```python
from build123d import *

# Parameters (mm, degrees)
SALIENTE_EXTRUIR1_DEPTH = 8
CORTAR_EXTRUIR1_DEPTH   = 10


with BuildPart() as part:
    # Croquis2 → Saliente-Extruir1 (new body)
    with BuildSketch(Plane.XY):
        with BuildLine():
            Line((614.835603051, 709.114300051), (830.835603051, 709.114300051))
            ThreePointArc((830.835603051, 709.114300051), (835.078243738, 710.871659363), (836.835603051, 715.114300051))
            Line((836.835603051, 715.114300051), (836.835603051, 819.114300051))
            ThreePointArc((836.835603051, 819.114300051), (835.078243738, 823.356940738), (830.835603051, 825.114300051))
            Line((830.835603051, 825.114300051), (614.835603051, 825.114300051))
            ThreePointArc((614.835603051, 825.114300051), (610.592962364, 823.356940738), (608.835603051, 819.114300051))
            Line((608.835603051, 819.114300051), (608.835603051, 715.114300051))
            ThreePointArc((608.835603051, 715.114300051), (610.592962364, 710.871659363), (614.835603051, 709.114300051))
        make_face()
    extrude(amount=SALIENTE_EXTRUIR1_DEPTH)

    # Croquis3 → Cortar-Extruir1 (cut)
    with BuildSketch(Plane(origin=(0, 0, 0), x_dir=(-1, 0, 0), z_dir=(0, 0, -1))):
        with BuildLine():
            Line((-616.135603051, 744.614300051), (-616.035603051, 744.614300051))
            ThreePointArc((-616.035603051, 744.614300051), (-614.479968132, 745.258665132), (-613.835603051, 746.814300051))
            Line((-613.835603051, 746.814300051), (-613.835603051, 787.414300051))
            ThreePointArc((-613.835603051, 787.414300051), (-614.479968132, 788.969934969), (-616.035603051, 789.614300051))
            Line((-616.035603051, 789.614300051), (-616.135603051, 789.614300051))
            ThreePointArc((-616.135603051, 789.614300051), (-617.691237969, 788.969934969), (-618.335603051, 787.414300051))
            Line((-618.335603051, 787.414300051), (-618.335603051, 746.814300051))
            ThreePointArc((-618.335603051, 746.814300051), (-617.691237969, 745.258665132), (-616.135603051, 744.614300051))
        make_face()
        with BuildLine():
            Line((-829.535603051, 789.614300051), (-829.635603051, 789.614300051))
            ThreePointArc((-829.635603051, 789.614300051), (-831.191237969, 788.969934969), (-831.835603051, 787.414300051))
            Line((-831.835603051, 787.414300051), (-831.835603051, 746.814300051))
            ThreePointArc((-831.835603051, 746.814300051), (-831.191237969, 745.258665132), (-829.635603051, 744.614300051))
            Line((-829.635603051, 744.614300051), (-829.535603051, 744.614300051))
            ThreePointArc((-829.535603051, 744.614300051), (-827.979968132, 745.258665132), (-827.335603051, 746.814300051))
            Line((-827.335603051, 746.814300051), (-827.335603051, 787.414300051))
            ThreePointArc((-827.335603051, 787.414300051), (-827.979968132, 788.969934969), (-829.535603051, 789.614300051))
        make_face()
    extrude(amount=-CORTAR_EXTRUIR1_DEPTH, mode=Mode.SUBTRACT)


solid = part.part
```
Model file for the job. Use its own axes, mm. A direction names the side the tool comes from. Give positions to 0.01 mm unless a question says otherwise; leave off trailing zeros. Write each loop counter-clockwise with the first axis right and the second up, starting at its lowest first coordinate (ties: lowest second). Pieces come first, ordered by that corner, then holes. Notation, with made-up numbers: (-38.75, 32) - (-7.75, 32) arc R25 cw to (-7.75, 53) - close; hole circle Ø2 at (35.5, 74). An arc over 180 degrees is marked (long way). One line per question, with ' | ' between items. Start each with the question number.
(1) Wall check: line 1 along X through (y, z) = (765, 4); line 2 along X through (y, z) = (746.5, 7.75); line 3 along Y through (x, z) = (828, 3.5). Give the ranges that are in metal, low to high. Write a range as from..to.
(2) Slice it at A-A on z = 3.5. Write the cut outline in (x, y).
(3) Two-plate mould, pull along X, no slides. Class faces 1 (the face through (831.836, 767, 4)), 2 (the face through (724, 825.114, 4)), 3 (the face through (608.836, 768, 4)), 4 (the face through (835.031, 710.825, 3.944)): +X half, -X half, draft (parallel to the pull), parting line (faces both ways), or undercut.
(4) 3-axis set-ups, long thin cutter, end or side, ignore diameter. For faces 5 (the face through (613.836, 767, 4)), 6 (the face through (721, 709.114, 4)): which of +Z, -Z, +X, -X, +Y, -Y reach the whole face in a straight line?
(5) Slice it at B-B on y = 759. Write the cut outline in (x, z), plus the area to 3 significant figures.
Results below:
1) line 1: 608.84..613.84, 618.34..827.34, 831.84..836.84 | line 2: 608.84..613.86, 618.31..827.36, 831.81..836.84 | line 3: 709.11..745.24, 788.99..825.11
2) outline: (608.84, 715.11) arc R6 ccw to (614.84, 709.11) - (830.84, 709.11) arc R6 ccw to (836.84, 715.11) - (836.84, 819.11) arc R6 ccw to (830.84, 825.11) - (614.84, 825.11) arc R6 ccw to (608.84, 819.11) - close; hole (613.84, 746.81) arc R2.2 ccw to (616.04, 744.61) - (616.14, 744.61) arc R2.2 ccw to (618.34, 746.81) - (618.34, 787.41) arc R2.2 ccw to (616.14, 789.61) - (616.04, 789.61) arc R2.2 ccw to (613.84, 787.41) - close; hole (827.34, 746.81) arc R2.2 ccw to (829.54, 744.61) - (829.64, 744.61) arc R2.2 ccw to (831.84, 746.81) - (831.84, 787.41) arc R2.2 ccw to (829.64, 789.61) - (829.54, 789.61) arc R2.2 ccw to (827.34, 787.41) - close
3) face 1: undercut | face 2: draft | face 3: -X half | face 4: +X half
4) face 5: +Z, -Z | face 6: +Z, -Z, +X, -X, -Y
5) outline: (608.84, 0) - (613.84, 0) - (613.84, 8) - (608.84, 8) - close; (618.34, 0) - (827.34, 0) - (827.34, 8) - (618.34, 8) - close; (831.84, 0) - (836.84, 0) - (836.84, 8) - (831.84, 8) - close | area: 1,750 mm^2
